```python
from build123d import *

# Parameters (mm, degrees)
BOSS_EXTRUDE1_START = -7.62
SKETCH2_R           = 35.56
BOSS_EXTRUDE1_DEPTH = 7.62
SKETCH4_R           = 8.89
SKETCH4_R_2         = 6.35
CUT_EXTRUDE1_REACH  = 157.543
SKETCH7_R           = 6.35
CUT_EXTRUDE2_REACH  = 147.358
SKETCH8_R           = 6.35
FILLET1_R           = 5.08


with BuildPart() as part:
    # Sketch1 → Revolve2 (revolve)
    with BuildSketch(Plane.XY, mode=Mode.PRIVATE) as revolve2_sk:
        Polygon((0, 0), (63.5, 0), (63.5, 76.2), (48.26, 76.2), (48.26, 127), (35.56, 127), (35.56, 63.5), (50.8, 63.5), (50.8, 12.7), (0, 12.7), align=None)
    revolve(revolve2_sk.sketch.rotate(Axis((0, 12.7, 0), (0, -1, 0)), 90), axis=Axis((0, 12.7, 0), (0, -1, 0)))

    # Sketch2 → Boss-Extrude1 (add)
    with BuildSketch(Plane(origin=(0, 114.3, 0), x_dir=(1, 0, 0), z_dir=(0, 1, 0)).offset(BOSS_EXTRUDE1_START)):
        with Locations(Location((0, 0, 0), (0, 0, 270))):
            Circle(SKETCH2_R)
    extrude(amount=BOSS_EXTRUDE1_DEPTH)

    # Sweep1: sweep along a path in Sketch5
    with BuildLine(Plane.XY) as sweep1_path:
        Line((15.24, 114.3), (15.24, 50.8))
        Line((15.24, 50.8), (33.02, 50.8))
        Line((33.02, 50.8), (33.02, 0))
    # Sketch4 → Sweep1 (sweep)
    with BuildSketch(Plane(origin=(0, 114.3, 0), x_dir=(1, 0, 0), z_dir=(0, 1, 0))):
        with Locations((15.24, 0)):
            Circle(SKETCH4_R)
        with Locations((15.24, 0)):
            Circle(SKETCH4_R_2, mode=Mode.SUBTRACT)
    sweep1 = sweep(path=sweep1_path.line, transition=Transition.RIGHT)

    # Sketch7 → Cut-Extrude1 (cut, up to next)
    with BuildSketch(Plane.XZ, mode=Mode.PRIVATE) as cut_extrude1_sk1:
        with Locations(Location((33.02, 0, 0), (0, 0, 270))):
            Circle(SKETCH7_R)
    cut_extrude1_tool1 = extrude(cut_extrude1_sk1.sketch, amount=-CUT_EXTRUDE1_REACH, mode=Mode.PRIVATE) & part.part
    cut_extrude1 = cut_extrude1_tool1.solids().sort_by_distance((33.02, 0, 0))[0]
    add(cut_extrude1, mode=Mode.SUBTRACT)

    # Sketch8 → Cut-Extrude2 (cut, up to next)
    with BuildSketch(Plane(origin=(0, 114.3, 0), x_dir=(1, 0, 0), z_dir=(0, 1, 0)), mode=Mode.PRIVATE) as cut_extrude2_sk1:
        with Locations(Location((15.24, 0, 0), (0, 0, 270))):
            Circle(SKETCH8_R)
    cut_extrude2_tool1 = extrude(cut_extrude2_sk1.sketch, amount=-CUT_EXTRUDE2_REACH, mode=Mode.PRIVATE) & part.part
    cut_extrude2 = cut_extrude2_tool1.solids().sort_by_distance((15.24, 114.3, 0))[0]
    add(cut_extrude2, mode=Mode.SUBTRACT)

    # Mirror1: Sweep1, Cut-Extrude1, Cut-Extrude2 across plane
    add(sweep1.mirror(Plane(origin=(0, 0, 0), x_dir=(0, 0, 1), z_dir=(1, 0, 0))))
    add(cut_extrude1.mirror(Plane(origin=(0, 0, 0), x_dir=(0, 0, 1), z_dir=(1, 0, 0))), mode=Mode.SUBTRACT)
    add(cut_extrude2.mirror(Plane(origin=(0, 0, 0), x_dir=(0, 0, 1), z_dir=(1, 0, 0))), mode=Mode.SUBTRACT)

    # Fillet1
    fillet1_edges = [part.edges().sort_by_distance(p)[0] for p in [
        (0, 76.2, -48.26),
        (0, 114.3, -35.56),
    ]]
    fillet(fillet1_edges, radius=FILLET1_R)


solid = part.part
```
Work out the finished part from the listing and answer in its coordinate system (mm). A direction names the side the tool comes from. Coordinates: 2 decimals unless noted, no trailing zeros. Write each loop counter-clockwise with the first axis right and the second up, starting at its lowest first coordinate (ties: lowest second). Pieces come first, ordered by that corner, then holes.
Q1. Which of the six approach directions +Z, -Z, +X, -X, +Y, -Y give full straight-line access (tool end or side, diameter ignored) to faces 1 (the face through (11.317, 79.864, 4.994)), 2 (the face through (-1, 12.7, -1))?
Q2. Find the intervals of material crossed by line 1 (X direction, y = 96.5, z = -0.5); line 2 (X direction, y = 36.5, z = 0); line 3 (Y direction, x = -28, z = 0), in increasing order.
Q3. A cutting plane is placed at B-B, the plane z = 0. State how many separate pieces and enclosed holes the cut face has, then the cut area to 3 significant figures.
Q4. A cutting plane is placed at A-A, the plane y = 89.5. Give the vertices of the cut face in (x, z), then the cut area to 3 significant figures.
Q5. Determine the mould class of faces 3 (the face through (-52, 76.2, -14)), 4 (the face through (41.232, 30.645, -3.405)) for opening direction X: released by +X, released by -X, zero draft, split by the parting line, or undercut.
Q6. A cutting plane is placed at C-C, the plane y = 47. Give the vertices of the cut face in (x, z).
Q7. Each of these flat-tipped pins is pushed along its axis until it touches: pin 1 Ø4 at (x, y) = (11, 22) entering from +Z; pin 2 Ø6 at (y, z) = (56.5, -34) entering from +X; pin 3 Ø18.5 at (x, z) = (-9, -3.5) entering from +Y. Where does it stop, or does it pass through?
Q8. A cutting plane is placed at D-D, the plane y = 31.5. Give the vertices of the cut face in (x, z).
Findings below:
1. face 1: +Y
1. face 2: none
2. line 1: x = -48.26 to -35.56, -24.12 to -21.57, -8.91 to -6.36, 6.36 to 8.91, 21.57 to 24.12, 35.56 to 48.26
2. line 2: x = -63.5 to -50.8, -41.91 to -39.37, -26.67 to -24.13, 24.13 to 26.67, 39.37 to 41.91, 50.8 to 63.5
2. line 3: y = 57.15 to 59.69, 106.68 to 114.3
3. separate pieces: 3
3. enclosed holes: 3
3. area: 6,090 mm2
4. outline: circle Ø96.52 at (0, 0); circle Ø17.78 at (-15.24, 0); circle Ø17.78 at (15.24, 0); hole circle Ø71.12 at (0, 0); hole circle Ø12.7 at (-15.24, 0); hole circle Ø12.7 at (15.24, 0)
4. area: 3,590 mm2
5. face 3: zero draft
5. face 4: undercut
6. outline: circle Ø127 at (0, 0); (-29.22, -8.04) - (-11.44, -8.04) arc R8.89 ccw to (-11.44, 8.04) - (-29.22, 8.04) arc R8.89 ccw (long way) to start; (11.44, -8.04) - (29.22, -8.04) arc R8.89 ccw (long way) to (29.22, 8.04) - (11.44, 8.04) arc R8.89 ccw to start; hole circle Ø101.6 at (0, 0); hole (-29.22, -5.09) - (-11.44, -5.09) arc R6.35 ccw to (-11.44, 5.09) - (-29.22, 5.09) arc R6.35 ccw (long way) to start; hole (11.44, -5.09) - (29.22, -5.09) arc R6.35 ccw (long way) to (29.22, 5.09) - (11.44, 5.09) arc R6.35 ccw to start
7. pin 1: stops at z = 62.86
7. pin 2: stops at x = 55.42
7. pin 3: stops at y = 114.3
8. outline: circle Ø127 at (0, 0); circle Ø17.78 at (-33.02, 0); circle Ø17.78 at (33.02, 0); hole circle Ø101.6 at (0, 0); hole circle Ø12.7 at (-33.02, 0); hole circle Ø12.7 at (33.02, 0)
